Study the drawing (mm; zero at the part's minimum x, y, z) and answer. Give positions to 0.01 mm unless a question says otherwise; leave off trailing zeros. Loops run counter-clockwise (first coordinate to the right, second up) from the corner with the lowest first, then second, coordinate; pieces in that order, holes last. Notation, with made-up numbers: M 2,-14.5 L 40,-14.5 A12 cw 40,-6.5 Z; hole C 61.5,84.5 d8. An arc over 180 degrees is marked long. Use one line per item in the form item = value. Start each with the question number.
1. This flat-tipped pin is pushed along its axis until it touches: pin 1 Ø2.5 at (x, z) = (71, 9) entering from -Y. Where does it stop, or does it pass through?
2. The part is cut by section C-C (y = 0.8). Write down the section's boundary in (x, z).
3. The part is cut by section A-A (x = 12). Write down the section's boundary in (y, z).
4. The part is cut by section D-D (x = 71). Write down the section's boundary in (y, z).
5. The part is cut by section B-B (z = 9). Write down the section's boundary in (x, y), and give its area (3 significant figures).
6. Straight lines are drawn through the part: line 1 (X direction, y = 0.6, z = 9); line 2 (Z direction, x = 26, y = 0.75); line 3 (Z direction, x = 12.5, y = 0.4). For each, find the intervals that lie inside material, in ascending order. Write a range as from..to.
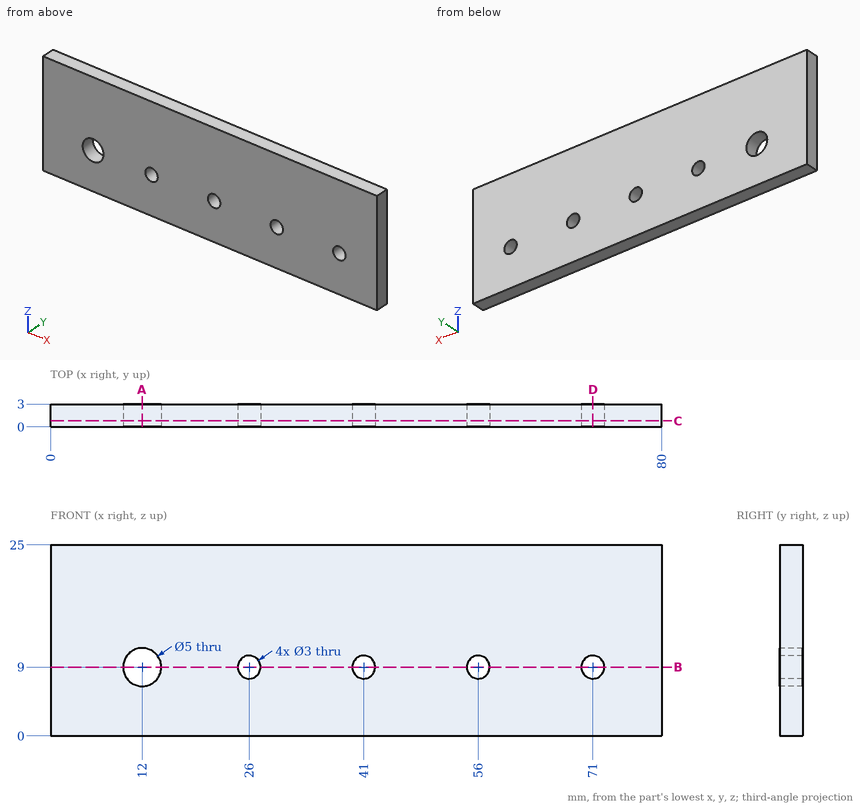
Derived:
q1.pin_1 = through
q2.outline = M 0,0 L 80,0 L 80,25 L 0,25 Z; hole C 12,9 d5; hole C 26,9 d3; hole C 41,9 d3; hole C 56,9 d3; hole C 71,9 d3
q3.outline = M 0,0 L 3,0 L 3,6.5 L 0,6.5 Z; M 0,11.5 L 3,11.5 L 3,25 L 0,25 Z
q4.outline = M 0,0 L 3,0 L 3,7.5 L 0,7.5 Z; M 0,10.5 L 3,10.5 L 3,25 L 0,25 Z
q5.outline = M 0,0 L 9.5,0 L 9.5,3 L 0,3 Z; M 14.5,0 L 24.5,0 L 24.5,3 L 14.5,3 Z; M 27.5,0 L 39.5,0 L 39.5,3 L 27.5,3 Z; M 42.5,0 L 54.5,0 L 54.5,3 L 42.5,3 Z; M 57.5,0 L 69.5,0 L 69.5,3 L 57.5,3 Z; M 72.5,0 L 80,0 L 80,3 L 72.5,3 Z
q5.area = 189 mm2
q6.line_1 = 0..9.5, 14.5..24.5, 27.5..39.5, 42.5..54.5, 57.5..69.5, 72.5..80
q6.line_2 = 0..7.5, 10.5..25
q6.line_3 = 0..6.55, 11.45..25
